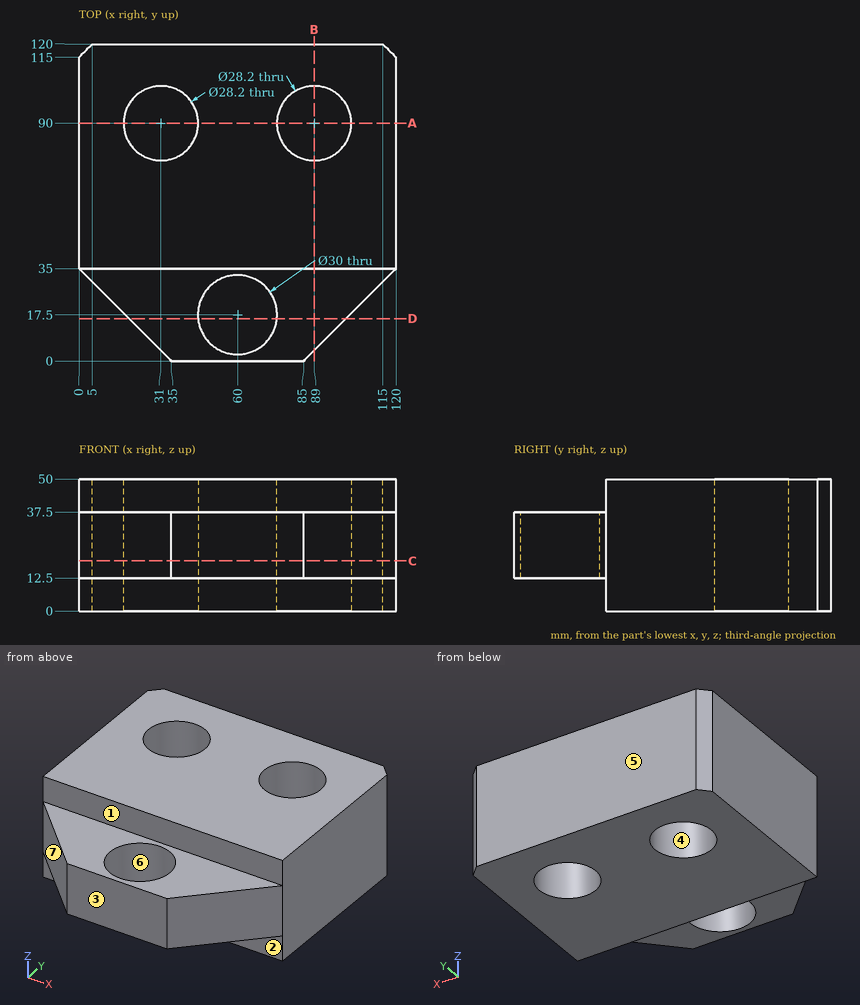
Source: three-view drawing plus pictorial views. Frame: mm from the lowest corner of the part. A direction names the side the tool comes from. Round coordinates to 2 decimals unless told otherwise and drop trailing zeros. Loops run counter-clockwise (first coordinate to the right, second up) from the corner with the lowest first, then second, coordinate; pieces in that order, holes last. Notation, with made-up numbers: (43, 79) - (91, 79) arc R12 ccw to (91, 99) - close; hole circle Ø2 at (2, 88.5). An arc over 180 degrees is marked (long way). Write item = value, one per line. Start each with the question number.
Item 1: Section query D-D on y = 16. Output: boundary loops of the cut face in (x, z), plus the area to 3 significant figures.
Item 2: Material intervals for line 1 (Y direction, x = 60, z = 32.25); line 2 (X direction, y = 102.5, z = 42); line 3 (X direction, y = 9, z = 15.5), sorted ascending.
Item 3: First-contact query: pin 1 Ø12 at (x, z) = (18, 31.5) entering from -Y; pin 2 Ø4 at (x, z) = (71, 41) entering from -Y; pin 3 Ø10.5 at (x, y) = (89, 11.5) entering from -Z; pin 4 Ø18 at (x, y) = (60, 17.5) entering from -Z. Flat tips, straight axial feed; report the tip coordinate or a pass-through.
Item 4: Section query A-A on y = 90. Output: boundary loops of the cut face in (x, z), plus the area to 3 significant figures.
Item 5: Section query B-B on x = 89. Output: boundary loops of the cut face in (y, z).
Item 6: Section query C-C on z = 19. Output: boundary loops of the cut face in (x, y).
Item 7: Reachability of the marked faces 1, 2 and 3 from +Z, -Z, +X, -X, +Y, -Y: full face, straight path, thin tool, end or side. Return the list, or none.
Item 8: Mould query, pull axis Y, two halves, no side actions, for the marked faces 4, 5, 6 and 7. Classes: released by +Y, released by -Y, zero draft, split by the parting line, or undercut.
Results list:
q1.outline = (19, 12.5) - (45.08, 12.5) - (45.08, 37.5) - (19, 37.5) - close; (74.92, 12.5) - (101, 12.5) - (101, 37.5) - (74.92, 37.5) - close
q1.area = 1,300 mm²
q2.line_1 = 0 to 2.5, 32.5 to 120
q2.line_2 = 0 to 24.48, 37.52 to 82.48, 95.52 to 120
q2.line_3 = 26 to 47.64, 72.36 to 94
q3.pin_1 = 11
q3.pin_2 = 35
q3.pin_3 = 12.5
q3.pin_4 = through
q4.outline = (0, 0) - (16.9, 0) - (16.9, 50) - (0, 50) - close; (45.1, 0) - (74.9, 0) - (74.9, 50) - (45.1, 50) - close; (103.1, 0) - (120, 0) - (120, 50) - (103.1, 50) - close
q4.area = 3,180 mm²
q5.outline = (4, 12.5) - (35, 12.5) - (35, 0) - (75.9, 0) - (75.9, 50) - (35, 50) - (35, 37.5) - (4, 37.5) - close; (104.1, 0) - (120, 0) - (120, 50) - (104.1, 50) - close
q6.outline = (0, 35) - (35, 0) - (85, 0) - (120, 35) - (120, 115) - (115, 120) - (5, 120) - (0, 115) - close; hole circle Ø28.2 at (31, 90); hole circle Ø30 at (60, 17.5); hole circle Ø28.2 at (89, 90)
q7.face_1 = +Z, +X, -X, -Y
q7.face_2 = -Z, +X, -X, -Y
q7.face_3 = +Z, -Z, +X, -X, -Y
q8.face_4 = undercut
q8.face_5 = released by +Y
q8.face_6 = undercut
q8.face_7 = released by -Y
